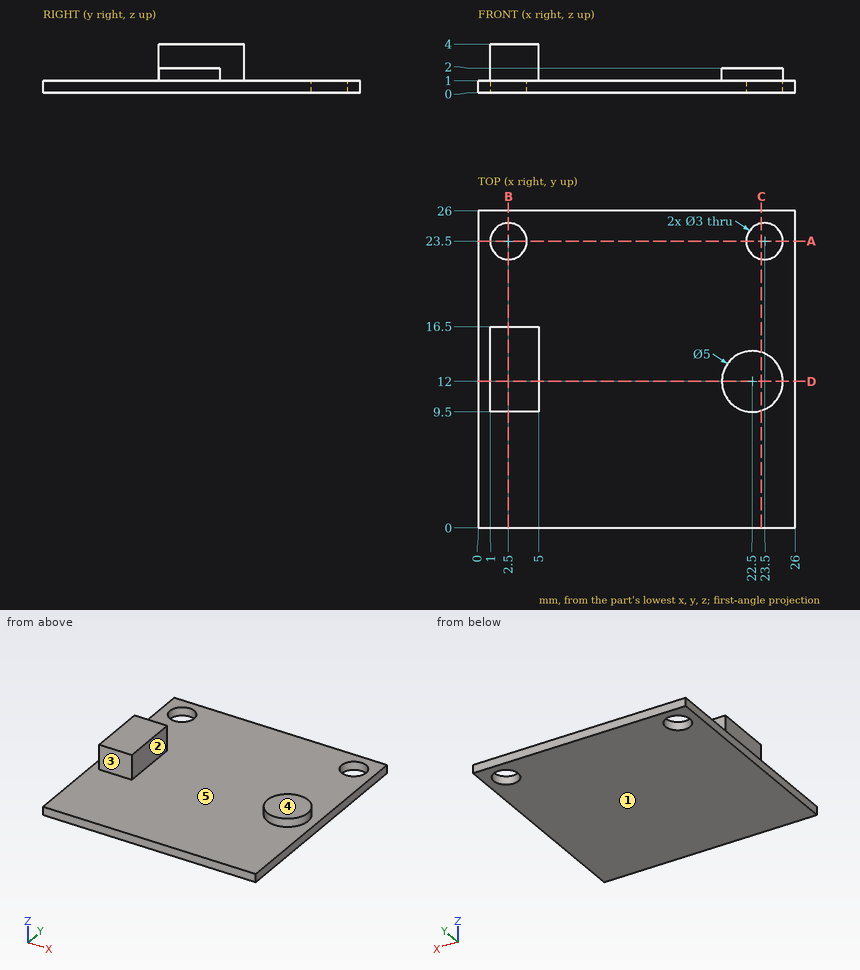
Could you check a few things on this drawing? It's one solid part, dimensions in mm from its lowest x, y, z. A direction names the side the tool comes from. Coordinates: 2 decimals unless noted, no trailing zeros. Write each loop counter-clockwise with the first axis right and the second up, starting at its lowest first coordinate (ties: lowest second). Pieces come first, ordered by that corner, then holes.
Q1. For P1, Ø0.9, axis at x = 3.5, z = 2, coming from the +Y side; P2, Ø8, axis at x = 7, y = 20, coming from the +Z side; P3, Ø2.5, axis at x = 2.5, y = 23.5, coming from the +Z side; P4, Ø4, axis at x = 23, y = 11, coming from the +Z side, each with a flat end and sliding along its axis, tell me the tip position at first contact or that it passes through.
Results found:
P1: stops at y = 16.5
P2: stops at z = 1
P3: passes through
P4: stops at z = 2
Q2. Imagine slicing it at B-B, the plane x = 2.5. List the corners of the cut face in (y, z) for me, plus the area to 3 significant figures.
Results found:
outline: (0, 0) - (22, 0) - (22, 1) - (16.5, 1) - (16.5, 4) - (9.5, 4) - (9.5, 1) - (0, 1) - close; (25, 0) - (26, 0) - (26, 1) - (25, 1) - close
area: 44.0 mm2
Q3. Imagine slicing it at C-C, the plane x = 23.25. List the corners of the cut face in (y, z) for me.
Results found:
outline: (0, 0) - (22.02, 0) - (22.02, 1) - (14.38, 1) - (14.38, 2) - (9.62, 2) - (9.62, 1) - (0, 1) - close; (24.98, 0) - (26, 0) - (26, 1) - (24.98, 1) - close
Q4. Please list where these lines run through material, in increasing order: L1, parallel to X at y = 23.5, z = 0.25; L2, parallel to Y at x = 23.5, z = 0.35; L3, parallel to X at y = 14.25, z = 3.
Results found:
L1: x = 0 to 1, 4 to 22, 25 to 26
L2: y = 0 to 22, 25 to 26
L3: x = 1 to 5
Q5. If we mould it in two halves opening along X, with no side actions, what happens to the marked faces 4 and 5? For each: +X half, -X half, draft (parallel to the pull), parting line (faces both ways), or undercut.
Results found:
face 4: draft
face 5: undercut
Q6. Imagine slicing it at A-A, the plane y = 23.5. List the corners of the cut face in (x, z) for me.
Results found:
outline: (0, 0) - (1, 0) - (1, 1) - (0, 1) - close; (4, 0) - (22, 0) - (22, 1) - (4, 1) - close; (25, 0) - (26, 0) - (26, 1) - (25, 1) - close
Q7. Imagine slicing it at D-D, the plane y = 12. List the corners of the cut face in (x, z) for me.
Results found:
outline: (0, 0) - (26, 0) - (26, 1) - (25, 1) - (25, 2) - (20, 2) - (20, 1) - (5, 1) - (5, 4) - (1, 4) - (1, 1) - (0, 1) - close
Q8. Which directions (+Z, -Z, +X, -X, +Y, -Y) give clear straight access to the entire face, cutting with the end or side of a thin tool? Please do the marked faces 1, 2 and 3.
Results found:
face 1: -Z, +X, -X, +Y, -Y
face 2: +Z, +Y, -Y
face 3: +Z, +X, -X, -Y
